```python
from build123d import *

# Parameters (mm, degrees)
SKETCH1_R           = 2.921
SKETCH1_R_2         = 1.0922
BOSS_EXTRUDE1_DEPTH = 9.525
FILLET1_R           = 7.62
CHAMFER1_SIZE       = 1.5875


with BuildPart() as part:
    # Sketch1 → Boss-Extrude1 (new body)
    with BuildSketch(Plane.XY):
        Polygon((0, 0), (54.714479363, -100.353454091), (54.714479363, 4.786896675), align=None)
        with Locations(Location((44.587010065, -55.247724238, 0), (0, 0, 180))):
            Circle(SKETCH1_R, mode=Mode.SUBTRACT)
        with Locations(Location((32.428236873, -32.946956662, 0), (0, 0, 180))):
            Circle(SKETCH1_R, mode=Mode.SUBTRACT)
        with Locations(Location((40.257483915, -0.047509878, 0), (0, 0, 180))):
            Circle(SKETCH1_R_2, mode=Mode.SUBTRACT)
        with Locations(Location((19.05, -12.35670409, 0), (0, 0, 180))):
            Circle(SKETCH1_R_2, mode=Mode.SUBTRACT)
    extrude(amount=BOSS_EXTRUDE1_DEPTH)

    # Fillet1
    fillet1_edges = [part.edges().sort_by_distance(p)[0] for p in [
        (54.714479363, 4.786896675, 4.7625),
        (54.714479363, -100.353454091, 4.7625),
        (0, 0, 4.7625),
    ]]
    fillet(fillet1_edges, radius=FILLET1_R)

    # Chamfer1
    chamfer1_edges = [part.edges().sort_by_distance(p)[0] for p in [
        (54.714479363, -36.993938617, 0),
        (54.714479363, -36.993938617, 9.525),
        (29.01531101, 2.538510782, 0),
        (22.989207497, -42.165189288, 0),
        (52.242476745, 2.089179203, 0),
        (5.548863872, -2.975274703, 0),
        (48.97661184, -77.842903003, 0),
        (22.989207497, -42.165189288, 9.525),
        (29.01531101, 2.538510782, 9.525),
        (52.242476745, 2.089179203, 9.525),
        (5.548863872, -2.975274703, 9.525),
        (48.97661184, -77.842903003, 9.525),
    ]]
    chamfer(chamfer1_edges, length=CHAMFER1_SIZE)


solid = part.part
```
Model file for the job. Use its own axes, mm. Coordinates: 2 decimals unless noted, no trailing zeros. Order: outer loops, then holes, each group sorted by start corner. A loop starts at its lowest first (then second) coordinate and runs counter-clockwise, first axis right, second up. Notation, with made-up numbers: (86, 76.25) - (118, 76.25) arc R21 ccw to (118, 103.25) - close; hole circle Ø1 at (-24.75, -35.75). An arc over 180 degrees is marked (long way). Return JSON: item names as keys, results as strings. Group by question number.
1) Saw through at C-C, the plane z = 6. Write the cut outline in (x, y), plus the area to 3 significant figures.
2) Flat gauge pins, fed straight in: P1, Ø5, axis at x = 22, z = 8.5, coming from the +Y side; P2, Ø4, axis at y = -17.5, z = 1, coming from the -X side; P3, Ø5, axis at x = 13, z = 7.5, coming from the -Y side. Where does each tip first touch, or does it go through?
3) Saw through at B-B, the plane y = -25. Write the cut outline in (x, z) (1 decimal).
4) Mould opens along X. For faces 1 (the flat face through (53.932, -37.462, 0.805)), 2 (the flat face through (23.43, -41.34, 8.72)), 3 (the cylindrical face through (39.216, -0.376, 4.696)) say: released by +X, released by -X, zero draft, split by the parting line, or undercut.
5) Saw through at A-A, the plane x = 19.05. Write the cut outline in (y, z) (1 decimal), plus the area to 3 significant figures.
6) Probe line 1 (Y direction, x = 30, z = 4.5); line 2 (Y direction, x = 19.05, z = 3); line 3 (X direction, y = -11.5, z = 3). List the from-to ranges inside material, lowest first. Write a range as from..to.
7) Saw through at D-D, the plane y = -51. Write the cut outline in (x, z) (1 decimal).
Values found:
{
 "1": {"outline": "(5.57, -10.22) - (40.4, -74.11) arc R7.62 ccw to (54.71, -70.46) - (54.71, -3.53) arc R7.62 ccw to (46.43, 4.06) - (11.6, 1.01) arc R7.62 ccw to start; hole circle Ø2.18 at (19.05, -12.36); hole circle Ø5.84 at (32.43, -32.95); hole circle Ø2.18 at (40.26, -0.05); hole circle Ø5.84 at (44.59, -55.25)", "area": "2,620 mm²"},
 "2": {"P1": "stops at y = 2.14", "P2": "stops at x = 8.5", "P3": "stops at y = -28.43"},
 "3": {"outline": "(13.6, 1.6) - (15.4, 0) - (53.1, 0) - (54.7, 1.6) - (54.7, 7.9) - (53.1, 9.5) - (15.4, 9.5) - (13.6, 7.9) - close"},
 "4": {"face 1": "released by +X", "face 2": "released by -X", "face 3": "undercut"},
 "5": {"outline": "(-34.9, 1.6) - (-31.6, 0) - (-13.4, 0) - (-13.4, 9.5) - (-31.6, 9.5) - (-34.9, 7.9) - close; (-11.3, 0) - (0.1, 0) - (1.7, 1.6) - (1.7, 7.9) - (0.1, 9.5) - (-11.3, 9.5) - close", "area": "320 mm²"},
 "6": {"line 1": "y = -55.02..-34.57, -31.32..2.62", "line 2": "y = -34.94..-13.45, -11.26..1.67", "line 3": "x = 6.27..18.37, 19.73..54.71"},
 "7": {"outline": "(27.8, 1.6) - (29.6, 0) - (53.1, 0) - (54.7, 1.6) - (54.7, 7.9) - (53.1, 9.5) - (29.6, 9.5) - (27.8, 7.9) - close"}
}
